Geometry check sheet. Reference: the model listing, model coordinates, mm. Round coordinates to 2 decimals unless told otherwise and drop trailing zeros. Order: outer loops, then holes, each group sorted by start corner. A loop starts at its lowest first (then second) coordinate and runs counter-clockwise, first axis right, second up. Notation, with made-up numbers: (-39.5, 64) - (2.5, 64) arc R25 ccw to (2.5, 88) - close; hole circle Ø10 at (-4.5, 24). An arc over 180 degrees is marked (long way). Use a Markdown table: item, result. Add a question column.
(1) Section check C-C on x = -9.5. Record the boundary of the cut face in (y, z), then the cut area to 4 significant figures.
(2) Gauge pin test, flat ends, axial feed: P1, Ø1.5, axis at y = 13, z = 1.5, coming from the -X side; P2, Ø1, axis at y = -2.5, z = 2, coming from the +X side. Record the tip position at first contact, or that the pin passes through.
(3) Section check D-D on y = 26. Record the boundary of the cut face in (x, z), then the cut area to 4 significant figures.
(4) Section check A-A on y = 0. Record the boundary of the cut face in (x, z).
(5) Section check B-B on z = 1.9. Record the boundary of the cut face in (x, y), then the cut area to 3 significant figures.
(6) Thickness scan on line 1 along X through (y, z) = (-10, 2.3); line 2 along Y through (x, z) = (-13.75, 2.05); line 3 along Y through (x, z) = (-2.5, 2.1). Record the ranges inside material, lowest first. Write a range as [from, to].
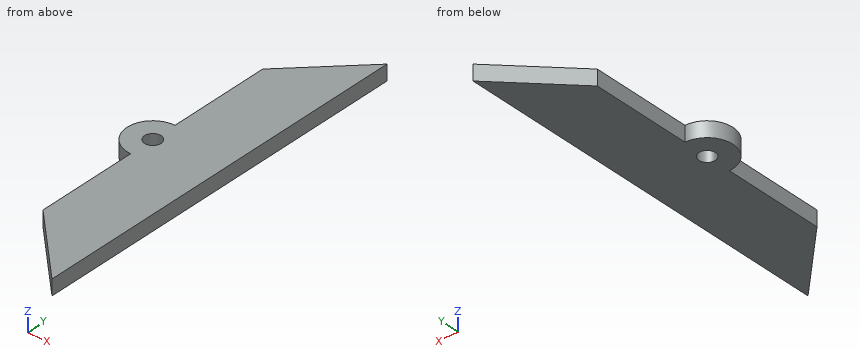
```python
from build123d import *

# Parameters (mm, degrees)
SKETCH1_R           = 5
BOSS_EXTRUDE1_DEPTH = 3
CUT_EXTRUDE1_REACH  = 43.929
SKETCH2_R           = 1.6


with BuildPart() as part:
    # Sketch1 → Boss-Extrude1 (new body)
    with BuildSketch(Plane.XY):
        with Locations((-13, 0)):
            Circle(SKETCH1_R)
        Polygon((-13, -24.75), (-13, 24.75), (0, 37.75), (0, -37.75), align=None)
    extrude(amount=BOSS_EXTRUDE1_DEPTH)

    # Sketch2 → Cut-Extrude1 (cut, up to next)
    with BuildSketch(Plane.XY.offset(3), mode=Mode.PRIVATE) as cut_extrude1_sk1:
        with Locations((-13, 0)):
            Circle(SKETCH2_R)
    cut_extrude1_tool1 = extrude(cut_extrude1_sk1.sketch, amount=-CUT_EXTRUDE1_REACH, mode=Mode.PRIVATE) & part.part
    add(cut_extrude1_tool1.solids().sort_by_distance((-13, 0, 3))[0], mode=Mode.SUBTRACT)


solid = part.part
```
Check sheet entries:
| question | item | result |
|---|---|---|
| 1 | outline | (-28.25, 0) - (28.25, 0) - (28.25, 3) - (-28.25, 3) - close |
| 1 | area | 169.5 mm2 |
| 2 | P1 | stops at x = -13 |
| 2 | P2 | stops at x = 0 |
| 3 | outline | (-11.75, 0) - (0, 0) - (0, 3) - (-11.75, 3) - close |
| 3 | area | 35.25 mm2 |
| 4 | outline | (-18, 0) - (-14.6, 0) - (-14.6, 3) - (-18, 3) - close; (-11.4, 0) - (0, 0) - (0, 3) - (-11.4, 3) - close |
| 5 | outline | (-13, -24.75) - (0, -37.75) - (0, 37.75) - (-13, 24.75) - (-13, 5) arc R5 ccw to (-13, -5) - close; hole circle Ø3.2 at (-13, 0) |
| 5 | area | 844 mm2 |
| 6 | line 1 | x = [-13, 0] |
| 6 | line 2 | y = [-4.94, -1.41], [1.41, 4.94] |
| 6 | line 3 | y = [-35.25, 35.25] |
